from build123d import *

# Parameters (mm, degrees)
SKETCH2_W                 = 95
SKETCH2_H                 = 95.25
BOSS_EXTRUDE3_DEPTH       = 4.7625
SKETCH3_R                 = 19.05
CUT_EXTRUDE1_DEPTH        = 77.928778953
M6X1_0_TAPPED_HOLE1_D     = 5
M6X1_0_TAPPED_HOLE1_DEPTH = 4.7625
M6X1_0_TAPPED_HOLE1_TIP   = 1.502151548
SKETCH7_R                 = 2.54
CUT_EXTRUDE2_DEPTH        = 7.62
SKETCH12_R                = 1.2446
CUT_EXTRUDE3_DEPTH        = 77.928778953


with BuildPart() as part:
    # Sketch2 → Boss-Extrude3 (new body)
    with BuildSketch(Plane(origin=(0, 0, 0), x_dir=(1, 0, 0), z_dir=(0, 1, 0))):
        with Locations((0, -12.7)):
            Rectangle(SKETCH2_W, SKETCH2_H)
    extrude(amount=BOSS_EXTRUDE3_DEPTH)

    # Sketch3 → Cut-Extrude1 (cut, through all)
    with BuildSketch(Plane(origin=(0, 4.7625, 0), x_dir=(1, 0, 0), z_dir=(0, 1, 0))):
        with Locations(Location((0, -22.225, 0), (0, 0, 270))):
            Circle(SKETCH3_R)
    extrude(amount=-CUT_EXTRUDE1_DEPTH, mode=Mode.SUBTRACT)

    # M6x1.0 Tapped Hole1
    with Locations(Plane(origin=(0, 4.7625, 0), x_dir=(1, 0, 0), z_dir=(0, 1, 0))):
        with Locations((-40, 19.685), (40, 19.685), (0, 19.685)):
            Hole(M6X1_0_TAPPED_HOLE1_D / 2, depth=M6X1_0_TAPPED_HOLE1_DEPTH)
            with Locations((0, 0, -(M6X1_0_TAPPED_HOLE1_DEPTH + M6X1_0_TAPPED_HOLE1_TIP / 2))):  # 118° drill point
                Cone(0, M6X1_0_TAPPED_HOLE1_D / 2, M6X1_0_TAPPED_HOLE1_TIP, mode=Mode.SUBTRACT)

    # Sketch7 → Cut-Extrude2 (cut)
    with BuildSketch(Plane(origin=(0, 4.7625, 0), x_dir=(1, 0, 0), z_dir=(0, 1, 0))):
        with Locations(Location((-33.02, -44.45, 0), (0, 0, 270))):
            Circle(SKETCH7_R)
        with Locations(Location((33.02, -44.45, 0), (0, 0, 270))):
            Circle(SKETCH7_R)
        with Locations(Location((-38.1, -52.07, 0), (0, 0, 270))):
            Circle(SKETCH7_R)
        with Locations(Location((38.1, -52.07, 0), (0, 0, 270))):
            Circle(SKETCH7_R)
    extrude(amount=-CUT_EXTRUDE2_DEPTH, mode=Mode.SUBTRACT)

    # Sketch12 → Cut-Extrude3 (cut, through all)
    with BuildSketch(Plane(origin=(0, 4.7625, 0), x_dir=(1, 0, 0), z_dir=(0, 1, 0))):
        with Locations(Location((0, 3.175, 0), (0, 0, 270))):
            Circle(SKETCH12_R)
        with Locations(Location((17.960512242, -4.264487758, 0), (0, 0, 270))):
            Circle(SKETCH12_R)
        with Locations(Location((25.4, -22.225, 0), (0, 0, 270))):
            Circle(SKETCH12_R)
        with Locations(Location((17.960512242, -40.185512242, 0), (0, 0, 270))):
            Circle(SKETCH12_R)
        with Locations(Location((0, -47.625, 0), (0, 0, 270))):
            Circle(SKETCH12_R)
        with Locations(Location((-17.960512242, -40.185512242, 0), (0, 0, 270))):
            Circle(SKETCH12_R)
        with Locations(Location((-25.4, -22.225, 0), (0, 0, 270))):
            Circle(SKETCH12_R)
        with Locations(Location((-17.960512242, -4.264487758, 0), (0, 0, 270))):
            Circle(SKETCH12_R)
    extrude(amount=-CUT_EXTRUDE3_DEPTH, mode=Mode.SUBTRACT)


solid = part.part
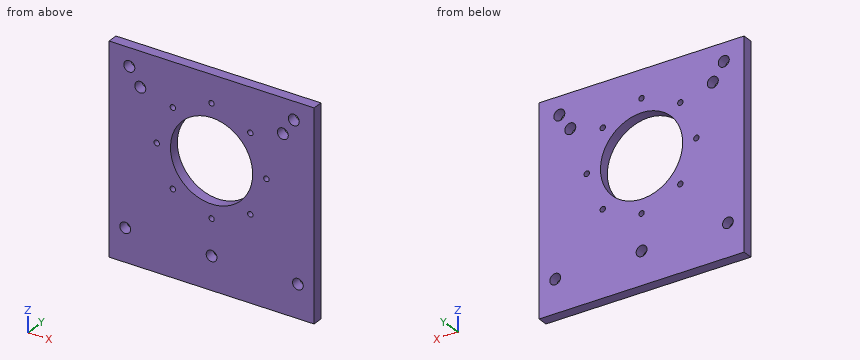
Read the model definition and answer for the solid it produces. Units are mm, in the model's axes. Give positions to 0.01 mm unless a question says otherwise; leave off trailing zeros. Write each loop counter-clockwise with the first axis right and the second up, starting at its lowest first coordinate (ties: lowest second). Pieces come first, ordered by that corner, then holes. Notation, with made-up numbers: (-25, 19) -> (16, 19) arc R20 ccw to (16, 53) -> close; hole circle Ø4 at (84, 16). An arc over 180 degrees is marked (long way). Answer as a JSON object with one key per item and string values. Group by question number.
1) Find section C-C (z = 14.5). Write down the section's boundary in (x, y), and give its area (3 significant figures).
2) Find section B-B (x = 25.4). Write down the section's boundary in (y, z) (1 decimal), and give its area (3 significant figures).
3) Find section A-A (z = 52.07). Write down the section's boundary in (x, y).
4) Consider L1, parallel to X at y = 3, z = 22; L2, parallel to X at y = 3.8, z = -21; L3, parallel to Z at x = -1, y = 2 (3 decimals). Determine where each line is inside the solid, lowest interval first. Write a range as from..to.
5) Find section D-D (y = 2.6). Count the separate pieces of the cut face and the enclosed holes in it, and give its area (3 significant figures).
Values follow:
{
 "1": {"outline": "(-47.5, 0) -> (-17.41, 0) -> (-17.41, 4.76) -> (-47.5, 4.76) -> close; (17.41, 0) -> (47.5, 0) -> (47.5, 4.76) -> (17.41, 4.76) -> close", "area": "287 mm2"},
 "2": {"outline": "(0, -34.9) -> (4.8, -34.9) -> (4.8, 21) -> (0, 21) -> close; (0, 23.5) -> (4.8, 23.5) -> (4.8, 60.3) -> (0, 60.3) -> close", "area": "442 mm2"},
 "3": {"outline": "(-47.5, 0) -> (-40.64, 0) -> (-40.64, 4.76) -> (-47.5, 4.76) -> close; (-35.56, 0) -> (35.56, 0) -> (35.56, 4.76) -> (-35.56, 4.76) -> close; (40.64, 0) -> (47.5, 0) -> (47.5, 4.76) -> (40.64, 4.76) -> close"},
 "4": {"L1": "x = -47.5..-26.62, -24.18..-19.05, 19.05..24.18, 26.62..47.5", "L2": "x = -47.5..-42.13, -37.87..-2.13, 2.13..37.87, 42.13..47.5", "L3": "z = -34.925..-21.976, -17.394..-3.916, -2.434..3.201, 41.249..46.884, 48.366..60.325"},
 "5": {"separate pieces": "1", "enclosed holes": "16", "area": "7,730 mm2"}
}
